Read the model definition and answer for the solid it produces. Units are mm, in the model's axes. A direction names the side the tool comes from. Coordinates: 2 decimals unless noted, no trailing zeros. Order: outer loops, then holes, each group sorted by start corner. A loop starts at its lowest first (then second) coordinate and runs counter-clockwise, first axis right, second up. Notation, with made-up numbers: (60.5, 14.5) - (82.5, 14.5) arc R17 cw to (82.5, 19.5) - close; hole circle Ø5 at (52.5, 26.25). An arc over 180 degrees is marked (long way). Write item = value, one per line.
from build123d import *

# Parameters (mm, degrees)
F0_W     = 65.991625
F0_H     = 80.656428
F1_DEPTH = 4
F3_R     = 10
F2_W     = 16.302
F2_H     = 5.422647
F4_DEPTH = 25


with BuildPart() as f1:
    # F0 (on Top) → F1 (new body)
    with BuildSketch(Plane.XY):
        with Locations((0.733241, -10.265363)):
            Rectangle(F0_W, F0_H)
    extrude(amount=F1_DEPTH)

    # F3
    f3_edges = [f1.edges().sort_by_distance(p)[0] for p in [
        (33.729054, 30.062851, 2),
        (-32.262571, 30.062851, 2),
        (-32.262571, -50.593577, 2),
        (33.729054, -50.593577, 2),
    ]]
    fillet(f3_edges, radius=F3_R)

    # F2 (on face) → F4 (cut)
    with BuildSketch(Plane.XY.offset(4)):
        with Locations((-0.79059, -41.648472)):
            Rectangle(F2_W, F2_H)
        Polygon((22.737429, 17.062851), (-21.262571, 17.062851), (-21.262571, -38.937149), (-8.94159, -38.937149), (7.36041, -38.937149), (22.737429, -38.937149), align=None)
    extrude(amount=-F4_DEPTH, mode=Mode.SUBTRACT)


solid = f1.part
1) The part is cut by section D-D (x = -27). Determine the outline of the cut face in (y, z).
Returned:
outline = (-49.4, 0) - (28.87, 0) - (28.87, 4) - (-49.4, 4) - close
2) Determine the mould class of faces 1 (the face through (30.877, 27.056, 2.028)), 2 (the face through (-22, -10, 4)), 3 (the face through (22.737, -11, 2)), 4 (the face through (-32.263, -11, 2)) for opening direction X: pulls with the +X half, pulls with the -X half, needs draft (parallel to the pull), parting line crosses it, or undercut.
Returned:
face_1 = pulls with the +X half
face_2 = needs draft
face_3 = undercut
face_4 = pulls with the -X half
3) The part is cut by section A-A (z = 1). Determine the outline of the cut face in (x, y), and give its area (3 significant figures).
Returned:
outline = (-32.26, -40.59) arc R10 ccw to (-22.26, -50.59) - (23.73, -50.59) arc R10 ccw to (33.73, -40.59) - (33.73, 20.06) arc R10 ccw to (23.73, 30.06) - (-22.26, 30.06) arc R10 ccw to (-32.26, 20.06) - close; hole (-21.26, -38.94) - (-8.94, -38.94) - (-8.94, -44.36) - (7.36, -44.36) - (7.36, -38.94) - (22.74, -38.94) - (22.74, 17.06) - (-21.26, 17.06) - close
area = 2,680 mm^2
4) The part is cut by section C-C (y = -7). Determine the outline of the cut face in (x, z), and give its area (3 significant figures).
Returned:
outline = (-32.26, 0) - (-21.26, 0) - (-21.26, 4) - (-32.26, 4) - close; (22.74, 0) - (33.73, 0) - (33.73, 4) - (22.74, 4) - close
area = 88.0 mm^2
5) Straight lines are drawn through the part: line 1 along X through (y, z) = (8.5, 2.25); line 2 along Y through (x, z) = (-5, 1.5); line 3 along Y through (x, z) = (8, 3.4). For each, find the intervals that lie inside material, in ascending order. Write a range as from..to.
Returned:
line_1 = -32.26..-21.26, 22.74..33.73
line_2 = -50.59..-44.36, 17.06..30.06
line_3 = -50.59..-38.94, 17.06..30.06
6) The part is cut by section B-B (x = -2.5). Determine the outline of the cut face in (y, z), and give its area (3 significant figures).
Returned:
outline = (-50.59, 0) - (-44.36, 0) - (-44.36, 4) - (-50.59, 4) - close; (17.06, 0) - (30.06, 0) - (30.06, 4) - (17.06, 4) - close
area = 76.9 mm^2
7) Flat-ended cylindrical pins translate along their axes: pin 1 Ø1 at (x, z) = (-25, 0.5) entering from -Y; pin 2 Ø12 at (x, y) = (12, 11) entering from +Z. Find the tip coordinate at first contact, or state that the pin passes through.
Returned:
pin_1 = -50.34
pin_2 = through
8) For faces 5 (the face through (-1, -44.36, 2)), 6 (the face through (-29.4, -47.6, 2)), determine the directions among +Z, -Z, +X, -X, +Y, -Y from which every point of the face is accessible in a straight line to the end or side of a thin tool.
Returned:
face_5 = +Z, -Z
face_6 = +Z, -Z, -X, -Y
